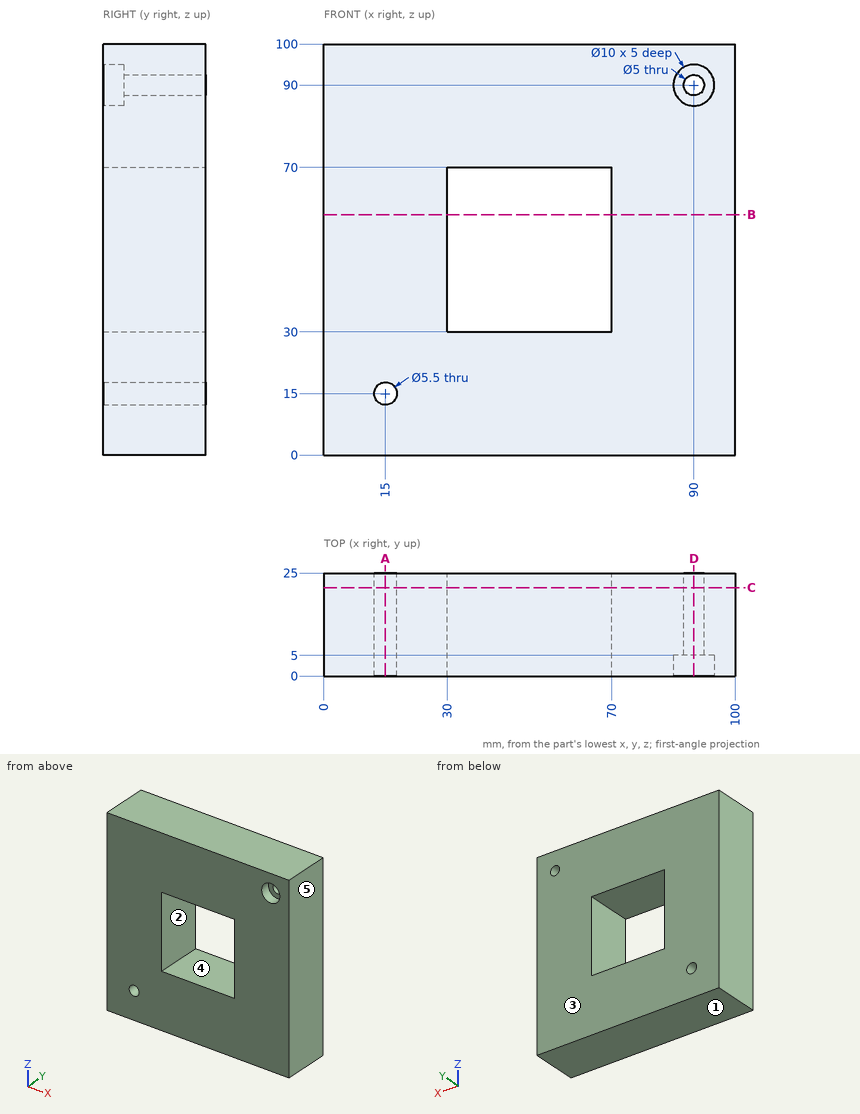
Can you work these out from the drawing? Everything is in mm from the part's minimum corner. A direction names the side the tool comes from. Round coordinates to 2 decimals unless told otherwise and drop trailing zeros. Write each loop counter-clockwise with the first axis right and the second up, starting at its lowest first coordinate (ties: lowest second). Pieces come first, ordered by that corner, then holes. Notation, with made-up numbers: M -19,80.5 L 37,80.5 A24 ccw 37,115.5 Z; hole C 34.5,43.5 d11. An arc over 180 degrees is marked long. Use a Markdown table: item, result.
Item 1: I want a section at D-D (x = 90). List the corners of the cut face in (y, z) for me, and give its area (3 significant figures).
Found:
| item | result |
|---|---|
| outline | M 0,0 L 25,0 L 25,87.5 L 5,87.5 L 5,85 L 0,85 Z; M 0,95 L 5,95 L 5,92.5 L 25,92.5 L 25,100 L 0,100 Z |
| area | 2,350 mm2 |
Item 2: We'd pull the mould along Z, two halves only. Please class the marked faces 1, 2 and 3: released by +Z, released by -Z, zero draft, split by the parting line, or undercut.
Found:
| item | result |
|---|---|
| face 1 | released by -Z |
| face 2 | undercut |
| face 3 | zero draft |
Item 3: Which directions (+Z, -Z, +X, -X, +Y, -Y) give clear straight access to the entire face, cutting with the end or side of a thin tool? Please do the marked faces 4 and 5.
Found:
| item | result |
|---|---|
| face 4 | +Y, -Y |
| face 5 | +Z, -Z, +X, +Y, -Y |
Item 4: I want a section at B-B (z = 58.5). List the corners of the cut face in (x, y) for me.
Found:
| item | result |
|---|---|
| outline | M 0,0 L 30,0 L 30,25 L 0,25 Z; M 70,0 L 100,0 L 100,25 L 70,25 Z |
Item 5: I want a section at A-A (x = 15). List the corners of the cut face in (y, z) for me.
Found:
| item | result |
|---|---|
| outline | M 0,0 L 25,0 L 25,12.25 L 0,12.25 Z; M 0,17.75 L 25,17.75 L 25,100 L 0,100 Z |
Item 6: If I drill on line 1 along Z through (x, y) = (90, 15.5); line 2 along X through (y, z) = (21.25, 48.5); line 3 along Z through (x, y) = (90, 1), over which ranges is the centre line in solid material (lowest first)? Write a range as [from, to].
Found:
| item | result |
|---|---|
| line 1 | z = [0, 87.5], [92.5, 100] |
| line 2 | x = [0, 30], [70, 100] |
| line 3 | z = [0, 85], [95, 100] |
Item 7: I want a section at C-C (y = 21.5). List the corners of the cut face in (x, z) for me.
Found:
| item | result |
|---|---|
| outline | M 0,0 L 100,0 L 100,100 L 0,100 Z; hole C 15,15 d5.5; hole M 30,30 L 70,30 L 70,70 L 30,70 Z; hole C 90,90 d5 |
